Check sheet for the modelled part. Datum: model origin and axes. Units: mm. A direction names the side the tool comes from. Round coordinates to 2 decimals unless told otherwise and drop trailing zeros. Loops run counter-clockwise (first coordinate to the right, second up) from the corner with the lowest first, then second, coordinate; pieces in that order, holes last. Notation, with made-up numbers: (81.25, 74.5) - (87.25, 74.5) arc R7 ccw to (87.25, 81.5) - close; hole circle Ø5 at (7, 30.5). An arc over 180 degrees is marked (long way). Put each result on its own line as item: value.
```python
from build123d import *

# Parameters (mm, degrees)
BOSS_EXTRUDE1_DEPTH = 4.826
CUT_EXTRUDE1_DEPTH  = 35.306
SKETCH3_R           = 3.048
CUT_EXTRUDE2_DEPTH  = 2.54
SKETCH4_R           = 1.778
SKETCH4_R_2         = 1.27
CUT_EXTRUDE3_DEPTH  = 5.826
CUT_EXTRUDE4_DEPTH  = 5.826


with BuildPart() as part:
    # Sketch1 → Boss-Extrude1 (new body)
    with BuildSketch(Plane.XY):
        with BuildLine():
            Line((0, 0), (-119.888, 0))
            Line((-119.888, 0), (-119.888, 12.7))
            Line((-119.888, 12.7), (-84.328, 12.7))
            ThreePointArc((-84.328, 12.7), (-82.531948776, 13.443948776), (-81.788, 15.24))
            Line((-81.788, 15.24), (-81.788, 19.05))
            Line((-81.788, 19.05), (0, 19.05))
            Line((0, 19.05), (0, 0))
        make_face()
    extrude(amount=BOSS_EXTRUDE1_DEPTH)

    # Sketch2 → Cut-Extrude1 (cut)
    with BuildSketch(Plane.ZY.offset(119.888)):
        Polygon((0.74979355, 12.7), (4.826, 8.258695089), (4.826, 12.7), align=None)
    extrude(amount=-CUT_EXTRUDE1_DEPTH, mode=Mode.SUBTRACT)

    # Sketch3 → Cut-Extrude2 (cut)
    with BuildSketch(Plane.XY.offset(4.826)):
        with Locations((-5.334, 9.525)):
            Circle(SKETCH3_R)
        with Locations((-84.328, 9.525)):
            Circle(SKETCH3_R)
    extrude(amount=-CUT_EXTRUDE2_DEPTH, mode=Mode.SUBTRACT)

    # Sketch4 → Cut-Extrude3 (cut, through all)
    with BuildSketch(Plane.XY.offset(4.826)):
        with Locations((-5.334, 9.525)):
            Circle(SKETCH4_R)
        with Locations((-84.328, 9.525)):
            Circle(SKETCH4_R)
        with Locations((-110.236, 5.588)):
            Circle(SKETCH4_R_2)
    extrude(amount=-CUT_EXTRUDE3_DEPTH, mode=Mode.SUBTRACT)

    # Sketch5 → Cut-Extrude4 (cut, through all)
    with BuildSketch(Plane.XY.offset(4.826)):
        with BuildLine():
            Line((-76.708, 12.741907021), (-13.0302, 12.741907021))
            ThreePointArc((-13.0302, 12.741907021), (-9.8933, 9.605007021), (-13.0302, 6.468107021))
            Line((-13.0302, 6.468107021), (-76.708, 6.468107021))
            ThreePointArc((-76.708, 6.468107021), (-79.8449, 9.605007021), (-76.708, 12.741907021))
        make_face()
    extrude(amount=-CUT_EXTRUDE4_DEPTH, mode=Mode.SUBTRACT)


solid = part.part
```
Item 1: Go/stop test with flat-tipped pins: pin 1 (4 mm diameter, centred on x = -84.328, y = 9.525, fed in from +Z); pin 2 (0.7 mm diameter, centred on y = 12, z = 2.5, fed in from -X); pin 3 (2.5 mm diameter, centred on x = -107, z = 2.5, fed in from +Y) (3 decimals). Record where each tip stops, or that it passes through.
Filled sheet:
pin 1: z = 2.29
pin 2: x = -84.58
pin 3: y = 12.155
Item 2: Release check for a two-part mould opening along Y. For faces 6 (the cylindrical face through (-82.552, 13.424, 2.379)), 7 (the flat face through (-59, 5, 4.826)), 8 (the cylindrical face through (-9.894, 9.674, 2.447)), 9 (the cylindrical face through (-82.78, 6.9, 3.57)) record: +Y half, -Y half, draft (parallel to the pull), parting line (faces both ways), or undercut.
Filled sheet:
face 6: +Y half
face 7: draft
face 8: undercut
face 9: undercut
Item 3: Section check C-C on x = -89. Enter the section's corners in (y, z).
Filled sheet:
outline: (0, 0) - (12.7, 0) - (12.7, 0.75) - (8.26, 4.83) - (0, 4.83) - close
Item 4: Section check B-B on z = 3.7. Enter the section's corners in (x, y) (3 decimals).
Filled sheet:
outline: (-119.888, 0) - (0, 0) - (0, 19.05) - (-81.788, 19.05) - (-81.788, 15.24) arc R2.54 cw to (-84.328, 12.7) - (-84.582, 12.7) - (-84.582, 12.562) arc R3.048 cw (long way) to (-87.376, 9.486) - (-119.888, 9.486) - close; hole circle Ø2.54 at (-110.236, 5.588); hole (-76.708, 6.468) - (-13.03, 6.468) arc R3.137 ccw to (-13.03, 12.742) - (-76.708, 12.742) arc R3.137 ccw to start; hole circle Ø6.096 at (-5.334, 9.525)
Item 5: Section check A-A on x = -44. Enter the section's corners in (y, z).
Filled sheet:
outline: (0, 0) - (6.47, 0) - (6.47, 4.83) - (0, 4.83) - close; (12.74, 0) - (19.05, 0) - (19.05, 4.83) - (12.74, 4.83) - close
Item 6: Tool access check on faces 1 (the flat face through (-45, 12.742, 2)), 2 (the flat face through (-41, 19.05, 2)), 3 (the flat face through (-4, 8, 2.286)), 4 (the flat face through (-102.2, 12.7, 0.3)), 5 (the flat face through (-102.48, 10.51, 2.76)). Record the directions out of +Z, -Z, +X, -X, +Y, -Y that give a thin tool (end or side, any length) a straight path to the whole face; none if there is none.
Filled sheet:
face 1: +Z, -Z
face 2: +Z, -Z, +X, -X, +Y
face 3: +Z
face 4: +Z, -Z, -X, +Y
face 5: +Z, -X, +Y
Item 7: Section check D-D on y = 17.5. Enter the section's corners in (x, z), then the cut area to 3 significant figures.
Filled sheet:
outline: (-81.79, 0) - (0, 0) - (0, 4.83) - (-81.79, 4.83) - close
area: 395 mm²
Item 8: Thickness scan on line 1 (Y direction, x = -45, z = 4.2); line 2 (X direction, y = 10.5, z = 2.8); line 3 (Y direction, x = -106, z = 0.6). Record the ranges inside material, lowest first. Write a range as from..to.
Filled sheet:
line 1: 0..6.47, 12.74..19.05
line 2: -81.44..-79.71, -10.02..-8.22, -2.45..0
line 3: 0..12.7
